The model under review builds one solid part; all positions refer to its coordinate system, in mm. A direction names the side the tool comes from. Round coordinates to 2 decimals unless told otherwise and drop trailing zeros. Loops run counter-clockwise (first coordinate to the right, second up) from the corner with the lowest first, then second, coordinate; pieces in that order, holes last. Notation, with made-up numbers: M 39.25,-4.75 L 97.25,-4.75 A22 ccw 97.25,7.25 Z; hole C 6.25,82.5 d5. An arc over 180 degrees is marked long. One line per question, with ' | ' between items.
from build123d import *

# Parameters (mm, degrees)
BOX009_W          = 12
BOX009_H          = 5
BOX009_DEPTH      = 10
BOX008_W          = 60
BOX008_H          = 22
BOX008_DEPTH      = 10
CYLINDER014_R     = 1.5
CYLINDER014_DEPTH = 20
CYLINDER013_R     = 1.5
CYLINDER013_DEPTH = 20
CYLINDER012_R     = 1.5
CYLINDER012_DEPTH = 20
CYLINDER015_R     = 1.5
CYLINDER015_DEPTH = 20
CYLINDER009_R     = 1.5
CYLINDER009_DEPTH = 20
CYLINDER010_R     = 1.5
CYLINDER010_DEPTH = 20
CYLINDER011_R     = 1.5
CYLINDER011_DEPTH = 20
CYLINDER008_R     = 1.5
CYLINDER008_DEPTH = 20
BOX003_W          = 92
BOX003_H          = 63
BOX003_DEPTH      = 2
FILLET001_R       = 6


with BuildPart() as cube006:
    # Box009 → Box009 (new body)
    with BuildSketch(Plane(origin=(68, 43, 20), x_dir=(1, 0, 0), z_dir=(0, 0, 1))):
        with Locations((6, 2.5)):
            Rectangle(BOX009_W, BOX009_H)
    extrude(amount=BOX009_DEPTH)


with BuildPart() as cube005:
    # Box008 → Box008 (new body)
    with BuildSketch(Plane(origin=(8.5, 38.5, 20), x_dir=(1, 0, 0), z_dir=(0, 0, 1))):
        with Locations((30, 11)):
            Rectangle(BOX008_W, BOX008_H)
    extrude(amount=BOX008_DEPTH)


with BuildPart() as cylinder014:
    # Cylinder014 → Cylinder014 (new body)
    with BuildSketch(Plane(origin=(82, 15.25, 20), x_dir=(1, 0, 0), z_dir=(0, 0, 1))):
        Circle(CYLINDER014_R)
    extrude(amount=CYLINDER014_DEPTH)


with BuildPart() as cylinder013:
    # Cylinder013 → Cylinder013 (new body)
    with BuildSketch(Plane(origin=(20, 15.25, 20), x_dir=(1, 0, 0), z_dir=(0, 0, 1))):
        Circle(CYLINDER013_R)
    extrude(amount=CYLINDER013_DEPTH)


with BuildPart() as cylinder012:
    # Cylinder012 → Cylinder012 (new body)
    with BuildSketch(Plane(origin=(2, 15.25, 20), x_dir=(1, 0, 0), z_dir=(0, 0, 1))):
        Circle(CYLINDER012_R)
    extrude(amount=CYLINDER012_DEPTH)


with BuildPart() as fusion003:
    # Cylinder015 → Cylinder015 (new body)
    with BuildSketch(Plane(origin=(62, 15.25, 20), x_dir=(1, 0, 0), z_dir=(0, 0, 1))):
        Circle(CYLINDER015_R)
    extrude(amount=CYLINDER015_DEPTH)

    # Fusion003: union Cylinder014, Cylinder013, Cylinder012
    add(cylinder014.part)
    add(cylinder013.part)
    add(cylinder012.part)


with BuildPart() as cylinder009:
    # Cylinder009 → Cylinder009 (new body)
    with BuildSketch(Plane(origin=(5.5, 9.25, 20), x_dir=(1, 0, 0), z_dir=(0, 0, 1))):
        Circle(CYLINDER009_R)
    extrude(amount=CYLINDER009_DEPTH)


with BuildPart() as cylinder010:
    # Cylinder010 → Cylinder010 (new body)
    with BuildSketch(Plane(origin=(5.5, 51.25, 20), x_dir=(1, 0, 0), z_dir=(0, 0, 1))):
        Circle(CYLINDER010_R)
    extrude(amount=CYLINDER010_DEPTH)


with BuildPart() as cylinder011:
    # Cylinder011 → Cylinder011 (new body)
    with BuildSketch(Plane(origin=(71.5, 54.25, 20), x_dir=(1, 0, 0), z_dir=(0, 0, 1))):
        Circle(CYLINDER011_R)
    extrude(amount=CYLINDER011_DEPTH)


with BuildPart() as fusion002:
    # Cylinder008 → Cylinder008 (new body)
    with BuildSketch(Plane(origin=(71.5, 6.25, 20), x_dir=(1, 0, 0), z_dir=(0, 0, 1))):
        Circle(CYLINDER008_R)
    extrude(amount=CYLINDER008_DEPTH)

    # Fusion002: union Cylinder009, Cylinder010, Cylinder011
    add(cylinder009.part)
    add(cylinder010.part)
    add(cylinder011.part)


with BuildPart() as middle_base:
    # Box003 → Box003 (new body)
    with BuildSketch(Plane(origin=(-2, -1, 0), x_dir=(1, 0, 0), z_dir=(0, 0, 1))):
        with Locations((46, 31.5)):
            Rectangle(BOX003_W, BOX003_H)
    extrude(amount=BOX003_DEPTH)

    # Fillet001
    fillet001_edges = [middle_base.edges().sort_by_distance(p)[0] for p in [
        (-2, -1, 1),
        (-2, 62, 1),
        (90, -1, 1),
        (90, 62, 1),
    ]]
    fillet(fillet001_edges, radius=FILLET001_R)


with BuildPart() as middle_base_1:
    # Fillet001 placement: moved
    add(middle_base.part.moved(Location((0, 0, 26))))

    # Cut002: cut Fusion002
    add(fusion002.part, mode=Mode.SUBTRACT)

    # Cut003: cut Fusion003
    add(fusion003.part, mode=Mode.SUBTRACT)

    # Cut007: cut Cube005
    add(cube005.part, mode=Mode.SUBTRACT)

    # Cut008: cut Cube006
    add(cube006.part, mode=Mode.SUBTRACT)


with BuildPart() as middle_base_2:
    # Cut008 placement: moved
    add(middle_base_1.part.moved(Location((0, 0, -6))))


solid = middle_base_2.part
1) Add section A-A on y = 51.25. State the section outline as (x, z) points, then the cut area to 3 significant figures.
Output values:
outline: M -2,20 L 4,20 L 4,22 L -2,22 Z; M 7,20 L 8.5,20 L 8.5,22 L 7,22 Z; M 68.5,20 L 90,20 L 90,22 L 68.5,22 Z | area: 58.0 mm²
2) Add section C-C on x = 44.5. State the section outline as (y, z) points.
Output values:
outline: M -1,20 L 38.5,20 L 38.5,22 L -1,22 Z; M 60.5,20 L 62,20 L 62,22 L 60.5,22 Z
3) Mouldability with a two-part tool opening along Y and no side actions: class faces 1 (the cylindrical face through (88.196, 0.711, 21.014)), 2 (the cylindrical face through (0.89, 16.26, 20.99)), 3 (the flat face through (-2, 30, 21)) as +Y half, -Y half, draft (parallel to the pull), parting line (faces both ways), or undercut.
Output values:
face 1: -Y half | face 2: undercut | face 3: draft
4) For line 1 (Y direction, x = 20, z = 20.7); line 2 (Y direction, x = 78.5, z = 21.6); line 3 (X direction, y = 44.5, z = 20.6), list the stretches that pass through material, from the lowest coordinate up.
Output values:
line 1: y = -1 to 13.75, 16.75 to 38.5, 60.5 to 62 | line 2: y = -1 to 43, 48 to 62 | line 3: x = -2 to 8.5, 80 to 90
5) Add section D-D on z = 21.4. State how many separate pieces and enclosed holes the cut face has, then the cut area to 3 significant figures.
Output values:
separate pieces: 1 | enclosed holes: 9 | area: 4,330 mm²
6) Machinability: for faces 4 (the flat face through (90, 30, 21)), 5 (the flat face through (74, 48, 21)), which of the approach directions +Z, -Z, +X, -X, +Y, -Y give a long, thin tool a straight path to every point of the face, cutting with its end or side? Answer none if there is none.
Output values:
face 4: +Z, -Z, +X, +Y, -Y | face 5: +Z, -Z
7) Add section B-B on x = 62. State the section outline as (y, z) points.
Output values:
outline: M -1,20 L 13.75,20 L 13.75,22 L -1,22 Z; M 16.75,20 L 38.5,20 L 38.5,22 L 16.75,22 Z; M 60.5,20 L 62,20 L 62,22 L 60.5,22 Z
